from build123d import *

# Parameters (mm, degrees)
SKETCH3_W                       = 19.05
SKETCH3_H                       = 44.45
BOSS_EXTRUDE1_DEPTH             = 457.2
BOSS_EXTRUDE1_DEPTH_BACK        = 457.2
FILLET1_R                       = 4.7625
SKETCH4_W                       = 447.675
SKETCH4_H                       = 44.45
CUT_EXTRUDE1_DEPTH              = 20.05
F_10_32_TAPPED_HOLE1_AT_2_COUNT = 2
F_10_32_TAPPED_HOLE1_AT_2_PITCH = 12.7
F_10_32_TAPPED_HOLE1_AT_3_COUNT = 2
F_10_32_TAPPED_HOLE1_AT_3_PITCH = 25.4
F_10_32_TAPPED_HOLE2_D          = 4.0386
F_10_32_TAPPED_HOLE2_DEPTH      = 9.525
F_10_32_TAPPED_HOLE2_TIP        = 1.213317848


with BuildPart() as part:
    # Sketch3 → Boss-Extrude1 (new body, two sides)
    with BuildSketch(Plane.XY) as boss_extrude1_sk:
        Rectangle(SKETCH3_W, SKETCH3_H)
    extrude(amount=BOSS_EXTRUDE1_DEPTH)
    extrude(boss_extrude1_sk.sketch, amount=-BOSS_EXTRUDE1_DEPTH_BACK)

    # Fillet1
    fillet1_edges = [part.edges().sort_by_distance(p)[0] for p in [
        (9.525, -22.225, 0),
        (-9.525, -22.225, 0),
        (-9.525, 22.225, 0),
        (9.525, 22.225, 0),
    ]]
    fillet(fillet1_edges, radius=FILLET1_R)

    # Sketch4 → Cut-Extrude1 (cut, through all)
    with BuildSketch(Plane(origin=(9.525, 0, 0), x_dir=(0, 0, -1), z_dir=(1, 0, 0))):
        with Locations((-233.3625, 0)):
            Rectangle(SKETCH4_W, SKETCH4_H)
        with Locations((233.3625, 0)):
            Rectangle(SKETCH4_W, SKETCH4_H)
    extrude(amount=-CUT_EXTRUDE1_DEPTH, mode=Mode.SUBTRACT)

    # Sketch6 → #10-32 Tapped Hole1 (revolve, cut)
    with BuildSketch(Plane(origin=(9.525, 12.7, -3.175), x_dir=(0, 0, -1), z_dir=(0, 1, 0))):
        Polygon((0, 0), (0, 10.738317848), (2.0193, 9.525), (2.0193, 0), align=None)
    f_10_32_tapped_hole1 = revolve(axis=Axis((15.875, 12.7, -3.175), (-1, 0, 0)), mode=Mode.SUBTRACT)

    # #10-32 Tapped Hole1 at 2: #10-32 Tapped Hole1 ×2
    with Locations(*[(0, -i * F_10_32_TAPPED_HOLE1_AT_2_PITCH, 0) for i in range(1, F_10_32_TAPPED_HOLE1_AT_2_COUNT)]):
        add(f_10_32_tapped_hole1, mode=Mode.SUBTRACT)

    # #10-32 Tapped Hole1 at 3: #10-32 Tapped Hole1 ×2
    with Locations(*[(0, -i * F_10_32_TAPPED_HOLE1_AT_3_PITCH, 0) for i in range(1, F_10_32_TAPPED_HOLE1_AT_3_COUNT)]):
        add(f_10_32_tapped_hole1, mode=Mode.SUBTRACT)

    # #10-32 Tapped Hole2
    with Locations(Plane.XY.offset(9.525)):
        with Locations((0, 0), (0, 12.7), (0, -12.7)):
            Hole(F_10_32_TAPPED_HOLE2_D / 2, depth=F_10_32_TAPPED_HOLE2_DEPTH)
            with Locations((0, 0, -(F_10_32_TAPPED_HOLE2_DEPTH + F_10_32_TAPPED_HOLE2_TIP / 2))):  # 118° drill point
                Cone(0, F_10_32_TAPPED_HOLE2_D / 2, F_10_32_TAPPED_HOLE2_TIP, mode=Mode.SUBTRACT)

    # Sketch12 → #10-32 Tapped Hole3 (revolve, cut)
    with BuildSketch(Plane(origin=(0, 22.225, -3.175), x_dir=(0, 0, 1), z_dir=(1, 0, 0))):
        Polygon((0, 0), (0, 10.738317848), (2.0193, 9.525), (2.0193, 0), align=None)
    f_10_32_tapped_hole3 = revolve(axis=Axis((0, 28.575, -3.175), (0, -1, 0)), mode=Mode.SUBTRACT)

    # Mirror1: #10-32 Tapped Hole3 across plane
    add(f_10_32_tapped_hole3.mirror(Plane.ZX), mode=Mode.SUBTRACT)

    # Mirror2: #10-32 Tapped Hole1 across plane
    add(f_10_32_tapped_hole1.mirror(Plane(origin=(0, 0, 0), x_dir=(0, 0, 1), z_dir=(1, 0, 0))), mode=Mode.SUBTRACT)

    # Mirror2 copy 1 sketch → Mirror2 copy 1 (revolve, cut)
    with BuildSketch(Plane(origin=(-9.525, 0, -3.175), x_dir=(0, 0, -1), z_dir=(0, 1, 0))):
        Polygon((0, 0), (0, -10.738317848), (2.0193, -9.525), (2.0193, 0), align=None)
    revolve(axis=Axis((-15.875, 0, -3.175), (-1, 0, 0)), mode=Mode.SUBTRACT)

    # Mirror2 copy 2 sketch → Mirror2 copy 2 (revolve, cut)
    with BuildSketch(Plane(origin=(-9.525, -12.7, -3.175), x_dir=(0, 0, -1), z_dir=(0, 1, 0))):
        Polygon((0, 0), (0, -10.738317848), (2.0193, -9.525), (2.0193, 0), align=None)
    revolve(axis=Axis((-15.875, -12.7, -3.175), (-1, 0, 0)), mode=Mode.SUBTRACT)


solid = part.part
The listing builds one solid part. Answer for the finished solid, in the listing's coordinates (mm). A direction names the side the tool comes from. Coordinates: 2 decimals unless noted, no trailing zeros. Loops run counter-clockwise (first coordinate to the right, second up) from the corner with the lowest first, then second, coordinate; pieces in that order, holes last. Notation, with made-up numbers: (-26, -39) -> (-3, -39) arc R23 ccw to (-3, -10) -> close; hole circle Ø7 at (9, 20.5). An arc over 180 degrees is marked (long way). Write item = value, one per line. Start each with the question number.
1) Given pin 1 Ø2.5 at (y, z) = (12.7, -3.175) entering from -X; pin 2 Ø3 at (x, z) = (0, -3.175) entering from +Y; pin 3 Ø2.5 at (x, y) = (0, 0) entering from +Z; pin 4 Ø3 at (x, y) = (0, -12.7) entering from +Z, each flat-ended and moving along its own axis, determine where each tip first touches the part or whether it passes through.
2) The mould has two halves that part along Z. Classify faces 1 (the face through (8.17, 20.79, -0.13)), 2 (the face through (2.3, -0.3, 9.525)), 3 (the face through (-0.13, 0.77, -5.04)): released by +Z, released by -Z, zero draft, split by the parting line, or undercut.
3) A cutting plane is placed at A-A (z = -4). Give the vertices of the cut face in (x, y) (1 decimal).
4) A cutting plane is placed at D-D (z = -6.25). Give the vertices of the cut face in (x, y) (1 decimal), then the cut area to 3 significant figures.
5) A cutting plane is placed at B-B (y = -16.5). Give the vertices of the cut face in (x, z) (3 decimals), then the cut area to 3 significant figures.
6) Straight lines are drawn through the part: line 1 (Y direction, x = -4.25, z = -3) (3 decimals); line 2 (X direction, y = 0, z = 5) (3 decimals); line 3 (Z direction, x = -6.75, y = 0) (3 decimals). For each, find the intervals that lie inside material, in ascending order. Write a range as from..to.
7) A tool of negligible diameter and unlimited length cuts with its end or side. For faces 4 (the face through (-0.089, -18.588, -5.192)), 5 (the face through (0.263, -10.698, 4.696)), 6 (the face through (-0.089, 18.588, -5.192)), from which of +Z, -Z, +X, -X, +Y, -Y can it reach the whole face along a straight path? Write none if from no direction.
8) A cutting plane is placed at C-C (z = 6.25). Give the vertices of the cut face in (x, y) (1 decimal), then the cut area to 3 significant figures.
Responses:
q1.pin_1 = through
q1.pin_2 = 11.35
q1.pin_3 = -0.46
q1.pin_4 = -0.31
q2.face_1 = zero draft
q2.face_2 = released by +Z
q2.face_3 = undercut
q3.outline = (-9.5, -17.5) arc R4.8 ccw to (-4.8, -22.2) -> (-1.8, -22.2) -> (-1.8, -14.5) -> (-9.5, -14.5) -> close; (-9.5, -10.9) -> (9.5, -10.9) -> (9.5, -1.8) -> (-9.5, -1.8) -> close; (-9.5, 1.8) -> (9.5, 1.8) -> (9.5, 10.9) -> (-9.5, 10.9) -> close; (-9.5, 14.5) -> (-1.8, 14.5) -> (-1.8, 22.2) -> (-4.8, 22.2) arc R4.8 ccw to (-9.5, 17.5) -> close; (1.8, -22.2) -> (4.8, -22.2) arc R4.8 ccw to (9.5, -17.5) -> (9.5, -14.5) -> (1.8, -14.5) -> close; (1.8, 14.5) -> (9.5, 14.5) -> (9.5, 17.5) arc R4.8 ccw to (4.8, 22.2) -> (1.8, 22.2) -> close
q4.outline = (-9.5, -17.5) arc R4.8 ccw to (-4.8, -22.2) -> (4.8, -22.2) arc R4.8 ccw to (9.5, -17.5) -> (9.5, 17.5) arc R4.8 ccw to (4.8, 22.2) -> (-4.8, 22.2) arc R4.8 ccw to (-9.5, 17.5) -> close
q4.area = 827 mm²
q5.outline = (-9.525, -9.525) -> (9.525, -9.525) -> (9.525, 9.525) -> (-9.525, 9.525) -> close; hole circle Ø4.039 at (0, -3.175)
q5.area = 350 mm²
q6.line_1 = -22.225..-14.712, -10.688..-2.012, 2.012..10.688, 14.712..22.225
q6.line_2 = -9.525..-2.019, 2.019..9.525
q6.line_3 = -9.525..-5.194, -1.156..9.525
q7.face_4 = -Y
q7.face_5 = +Z
q7.face_6 = +Y
q8.outline = (-9.5, -17.5) arc R4.8 ccw to (-4.8, -22.2) -> (4.8, -22.2) arc R4.8 ccw to (9.5, -17.5) -> (9.5, 17.5) arc R4.8 ccw to (4.8, 22.2) -> (-4.8, 22.2) arc R4.8 ccw to (-9.5, 17.5) -> close; hole circle Ø4 at (0, -12.7); hole circle Ø4 at (0, 0); hole circle Ø4 at (0, 12.7)
q8.area = 789 mm²
